Input: dimensioned drawing with shaded views. Units: mm. Origin: part minimum x, y, z. Coordinates: 2 decimals unless noted, no trailing zeros. Loops run counter-clockwise (first coordinate to the right, second up) from the corner with the lowest first, then second, coordinate; pieces in that order, holes last.
Item 1: Section query C-C, the plane y = 5.25. Return the cut outline in (x, z) (1 decimal), then the cut area to 3 significant figures.
Item 2: Line query: probe 1 along X at (y, z) = (1.5, 152.4); probe 2 along Z at (x, y) = (241.3, 1.75); probe 3 along Z at (x, y) = (55, 4.25) (1 decimal). Output: solid intervals per line, ascending.
Item 3: Section query D-D, the plane x = 12.7. Return the cut outline in (y, z), then the cut area to 3 significant figures.
Item 4: Section query A-A, the plane x = 241.3. Return the cut outline in (y, z), then the cut area to 3 significant figures.
Item 5: Section query B-B, the plane z = 203.2. Return the cut outline in (x, y), then the cut area to 3 significant figures.
Item 6: Pin query (flat end, axial travel): pin 1 Ø3 at (y, z) = (2.5, 314) entering from +X. Return the tip coordinate at first contact, or that it passes through.
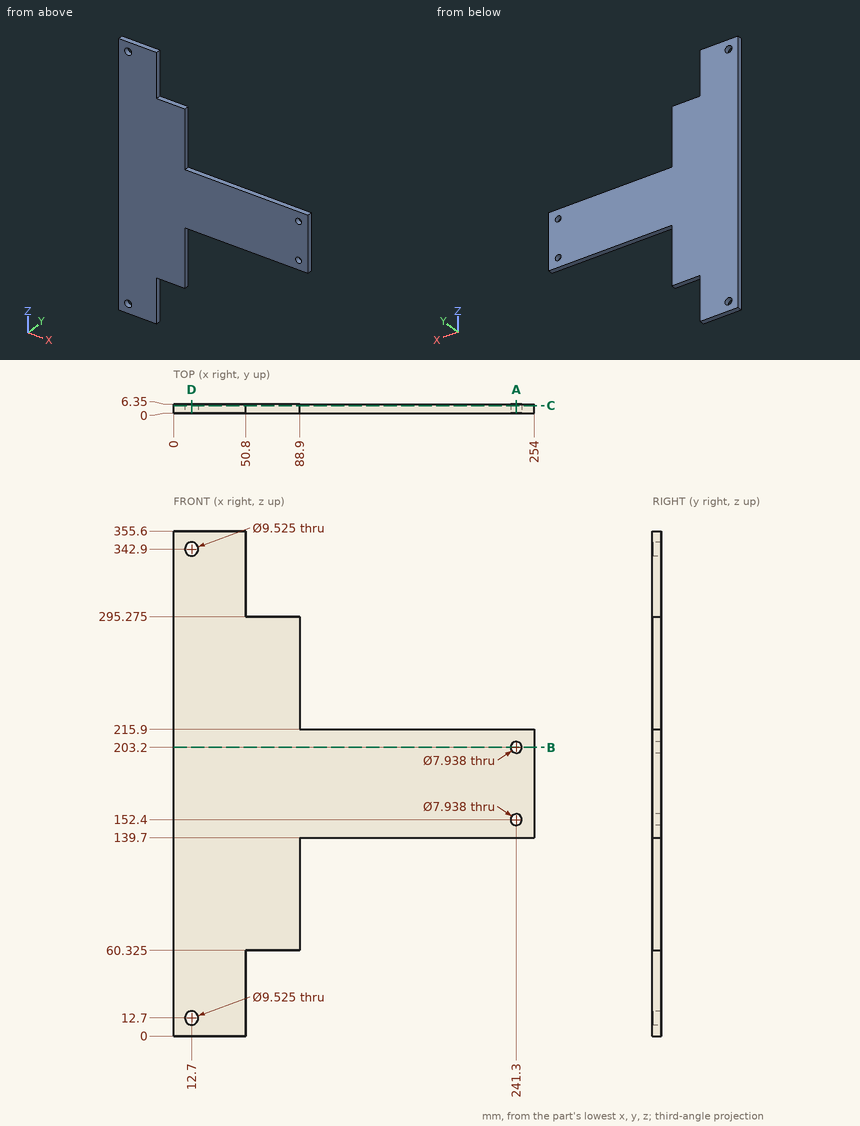
Verdict:
1. outline: (0, 0) - (50.8, 0) - (50.8, 60.3) - (88.9, 60.3) - (88.9, 139.7) - (254, 139.7) - (254, 215.9) - (88.9, 215.9) - (88.9, 295.3) - (50.8, 295.3) - (50.8, 355.6) - (0, 355.6) - close; hole circle Ø9.5 at (12.7, 12.7); hole circle Ø9.5 at (12.7, 342.9); hole circle Ø7.9 at (241.3, 152.4); hole circle Ø7.9 at (241.3, 203.2)
1. area: 39,400 mm2
2. probe 1: x = 0 to 237.33, 245.27 to 254
2. probe 2: z = 139.7 to 148.43, 156.37 to 199.23, 207.17 to 215.9
2. probe 3: z = 60.3 to 295.3
3. outline: (0, 0) - (6.35, 0) - (6.35, 7.94) - (0, 7.94) - close; (0, 17.46) - (6.35, 17.46) - (6.35, 338.14) - (0, 338.14) - close; (0, 347.66) - (6.35, 347.66) - (6.35, 355.6) - (0, 355.6) - close
3. area: 2,140 mm2
4. outline: (0, 139.7) - (6.35, 139.7) - (6.35, 148.43) - (0, 148.43) - close; (0, 156.37) - (6.35, 156.37) - (6.35, 199.23) - (0, 199.23) - close; (0, 207.17) - (6.35, 207.17) - (6.35, 215.9) - (0, 215.9) - close
4. area: 383 mm2
5. outline: (0, 0) - (237.33, 0) - (237.33, 6.35) - (0, 6.35) - close; (245.27, 0) - (254, 0) - (254, 6.35) - (245.27, 6.35) - close
5. area: 1,560 mm2
6. pin 1: stops at x = 50.8
